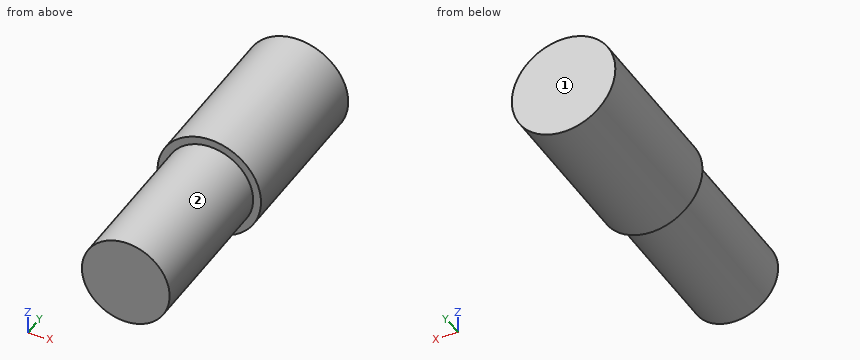
from build123d import *

# Parameters (mm, degrees)
F0_W     = 32.7049233019
F0_H     = 104.7131195664
F2_T     = -5
F3_DEPTH = 200


with BuildPart() as f1:
    # F0 (on Top) → F1 (revolve)
    with BuildSketch(Plane.XY):
        with Locations((-16.352461651, 0)):
            Rectangle(F0_W, F0_H)
    revolve(axis=Axis((0, 0, 0), (0, -1, 0)))

    # F2
    f2_openings = [f1.faces().sort_by_distance(p)[0] for p in [
        (0, -52.35656, 0),
    ]]
    offset(amount=F2_T, openings=f2_openings)

    # F3 (add): a face of the model
    f3_faces = [f1.faces().sort_by_distance(p)[0] for p in [
        (0, 47.3565597832, 0),
    ]]
    extrude(f3_faces, amount=F3_DEPTH)


solid = f1.part
Geometry: final body of the model. Coordinates: model frame, mm. Face numbers are marked on the shaded views. A direction names the side the tool comes from. Give positions to 0.01 mm unless a question says otherwise; leave off trailing zeros. Write each loop counter-clockwise with the first axis right and the second up, starting at its lowest first coordinate (ties: lowest second). Pieces come first, ordered by that corner, then holes.
(1) Cut plane C-C, the plane y = -16.5. Return loops of the section in (x, z).
(2) Cut plane A-A, the plane x = 0. Return loops of the section in (y, z), then the cut area to 3 significant figures.
(3) Ray query, line 1 (Z direction, x = -1.5, y = -129); line 2 (Y direction, x = 25.5, z = -13); line 3 (X direction, y = 18.5, z = -20). Return the intervals inside material, ascending.
(4) Access query for the marked faces 1 and 2. Directions: +Z, -Z, +X, -X, +Y, -Y. A direction counts if a zero-diameter tool reaches every point of the face in a straight line with its end or side. Return the directions, or none.
(5) Cut plane D-D, the plane y = -76.5. Return loops of the section in (x, z), then the cut area to 3 significant figures.
(6) First-contact query: P1, Ø3, axis at x = 12.5, y = -83.5, coming from the -Z side; P2, Ø4, axis at y = -14, z = -4.5, coming from the +X side; P3, Ø6, axis at x = 10, y = 7.5, coming from the +Z side. Flat tips, straight axial feed; report the tip coordinate or a pass-through.
(7) Cut plane B-B, the plane z = -14. Return loops of the section in (x, y).
Values follow:
1. outline: circle Ø65.41 at (0, 0)
2. outline: (-152.64, -27.7) - (-52.36, -27.7) - (-52.36, -32.7) - (52.36, -32.7) - (52.36, 32.7) - (-52.36, 32.7) - (-52.36, 27.7) - (-152.64, 27.7) - close
2. area: 12,400 mm2
3. line 1: z = -27.66 to 27.66
3. line 2: y = -52.36 to 52.36
3. line 3: x = -25.88 to 25.88
4. face 1: +Z, -Z, +X, -X, +Y
4. face 2: -Y
5. outline: circle Ø55.41 at (0, 0)
5. area: 2,410 mm2
6. P1: stops at z = -25.43
6. P2: stops at x = 32.61
6. P3: stops at z = 31.95
7. outline: (-29.56, -52.36) - (-23.91, -52.36) - (-23.91, -152.64) - (23.91, -152.64) - (23.91, -52.36) - (29.56, -52.36) - (29.56, 52.36) - (-29.56, 52.36) - close
